Geometry check sheet. Reference: the model listing, model coordinates, mm. A direction names the side the tool comes from. Give positions to 0.01 mm unless a question says otherwise; leave off trailing zeros. Write each loop counter-clockwise with the first axis right and the second up, starting at its lowest first coordinate (ties: lowest second). Pieces come first, ordered by that corner, then holes. Notation, with made-up numbers: M -31,66 L 12,66 A16 cw 12,85 Z; hole C -34,77 d11. An arc over 180 degrees is marked long. Write each question's results on one line, items separated by ' | '.
```python
from build123d import *

# Parameters (mm, degrees)
SKETCH2_R               = 7.5
BOSS_EXTRUDE1_DEPTH     = 4
SKETCH4_R               = 3.625
BOSS_EXTRUDE3_DEPTH     = 15
BOSS_EXTRUDE4_DEPTH     = 20
CUT_EXTRUDE1_DEPTH      = 23.638462845
CUT_EXTRUDE1_DEPTH_BACK = 23.638462845
SKETCH1_R               = 3
SKETCH6_R               = 0.75
CUT_EXTRUDE2_DEPTH      = 2
CIRPATTERN1_COUNT       = 3
MIRROR1_COPY_1_SKETCH_R = 0.75
MIRROR1_COPY_1_DEPTH    = 2
MIRROR1_COPY_2_SKETCH_R = 0.75
MIRROR1_COPY_2_DEPTH    = 2


with BuildPart() as part:
    # Sketch2 → Boss-Extrude1 (new, symmetric)
    with BuildSketch(Plane(origin=(0, 0, 0), x_dir=(0, 0, -1), z_dir=(1, 0, 0))):
        Circle(SKETCH2_R)
    extrude(amount=BOSS_EXTRUDE1_DEPTH, both=True)

    # Sketch4 → Boss-Extrude3 (add, symmetric)
    with BuildSketch(Plane(origin=(0, 0, 0), x_dir=(0, 0, -1), z_dir=(1, 0, 0))):
        Circle(SKETCH4_R)
    extrude(amount=BOSS_EXTRUDE3_DEPTH, both=True)

    # Sketch5 → Boss-Extrude4 (add, symmetric)
    with BuildSketch(Plane.ZY):
        Polygon((0, 3.625), (-3.139342089, 1.8125), (-3.139342089, -1.8125), (0, -3.625), (3.139342089, -1.8125), (3.139342089, 1.8125), align=None)
    extrude(amount=BOSS_EXTRUDE4_DEPTH, both=True)

    # Sketch1 → Cut-Extrude1 (cut, two sides: drawn at the far end of the back side and taken through both)
    with BuildSketch(Plane.XY.offset(-CUT_EXTRUDE1_DEPTH_BACK)):
        Circle(SKETCH1_R)
    extrude(amount=CUT_EXTRUDE1_DEPTH + CUT_EXTRUDE1_DEPTH_BACK, mode=Mode.SUBTRACT)

    # Sketch6 → Cut-Extrude2 (cut)
    with BuildSketch(Plane(origin=(0, 3.625, -26.115381057), x_dir=(-1, 0, 0), z_dir=(0, -1, 0))):
        with Locations(Location((17.5, -26.115381057, 0), (0, 0, 180))):
            Circle(SKETCH6_R)
    cut_extrude2 = extrude(amount=CUT_EXTRUDE2_DEPTH, mode=Mode.SUBTRACT)

    # CirPattern1: Cut-Extrude2 ×3 about axis
    cirpattern1_axis = Axis((0, 0, 0), (1, 0, 0))
    for i in range(1, CIRPATTERN1_COUNT):
        add(cut_extrude2.rotate(cirpattern1_axis, i * 360 / CIRPATTERN1_COUNT), mode=Mode.SUBTRACT)

    # Mirror1: Cut-Extrude2 across plane
    add(cut_extrude2.mirror(Plane(origin=(0, 0, 0), x_dir=(0, 0, 1), z_dir=(1, 0, 0))), mode=Mode.SUBTRACT)

    # Mirror1 copy 1 sketch → Mirror1 copy 1 (cut)
    with BuildSketch(Plane(origin=(0, 20.804083425, 16.197032617), x_dir=(1, 0, 0), z_dir=(0, 0.4999999999999998, -0.8660254037844387))):
        with Locations((17.5, 26.115381057)):
            Circle(MIRROR1_COPY_1_SKETCH_R)
    extrude(amount=MIRROR1_COPY_1_DEPTH, mode=Mode.SUBTRACT)

    # Mirror1 copy 2 sketch → Mirror1 copy 2 (cut)
    with BuildSketch(Plane(origin=(0, -24.429083425, 9.91834844), x_dir=(1, 0, 0), z_dir=(0, 0.5000000000000004, 0.8660254037844384))):
        with Locations((17.5, 26.115381057)):
            Circle(MIRROR1_COPY_2_SKETCH_R)
    extrude(amount=MIRROR1_COPY_2_DEPTH, mode=Mode.SUBTRACT)


solid = part.part
```
Q1. Section check A-A (y = 0.5). Enter the section's corners in (x, z).
Answer key:
outline: M -20,-3.14 L -15,-3.14 L -15,-3.59 L -4,-3.59 L -4,-7.48 L -2.96,-7.48 L -2.96,7.48 L -4,7.48 L -4,3.59 L -15,3.59 L -15,3.14 L -20,3.14 Z; M 2.96,-7.48 L 4,-7.48 L 4,-3.59 L 15,-3.59 L 15,-3.14 L 20,-3.14 L 20,3.14 L 15,3.14 L 15,3.59 L 4,3.59 L 4,7.48 L 2.96,7.48 Z
Q2. Release check for a two-part mould opening along X. For faces 4 (the face through (-18.25, -1.24, 2.08)), 5 (the face through (-4, 3.44, -1.56)), 6 (the face through (16.75, -1.18, -2.11)), 7 (the face through (15, 2.9, -1.7)) record: released by +X, released by -X, zero draft, split by the parting line, or undercut.
Answer key:
face 4: undercut | face 5: released by -X | face 6: undercut | face 7: released by +X
Q3. Material ranges on probe 1 along X at (y, z) = (0, 1); probe 2 along Z at (x, y) = (-17.5, 2.7); probe 3 along X at (y, z) = (-4.25, -5.25), recorded low to high. Write a range as [from, to].
Answer key:
probe 1: x = [-20, -3], [3, 20] | probe 2: z = [-1.6, -0.75], [0.75, 1.6] | probe 3: x = [-4, 4]
Q4. Section check D-D (y = 6). Enter the section's corners in (x, z), then the cut area to 3 significant figures.
Answer key:
outline: M -4,-4.5 L 4,-4.5 L 4,4.5 L -4,4.5 Z | area: 72.0 mm2
Q5. Section check B-B (z = 6). Enter the section's corners in (x, y), then the cut area to 3 significant figures.
Answer key:
outline: M -4,-4.5 L 4,-4.5 L 4,4.5 L -4,4.5 Z; hole C 0,0 d6 | area: 43.7 mm2
Q6. Depth check by flat-ended pin: P1, Ø1, axis at y = 3, z = -5, coming from the +X side; P2, Ø1.8, axis at x = 16.5, y = 0.5, coming from the +Z side; P3, Ø6, axis at x = -5.5, y = 3, coming from the -Z side. Enter the tip coordinate at first touch or a pass-through.
Answer key:
P1: stops at x = 4 | P2: stops at z = 3.14 | P3: stops at z = -7.49
Q7. Access from +Z, -Z, +X, -X, +Y, -Y to the whole of each face (thin tool, end or side, straight path). Record for faces 1 (the face through (18, 1.625, 0)), 2 (the face through (17.49, -0.803, -1.413)), 3 (the face through (17.46, -2.73, 1.55)).
Answer key:
face 1: +Y | face 2: none | face 3: +Z, +X, -Y
